Work out the finished part from the listing and answer in its coordinate system (mm). A direction names the side the tool comes from. Round coordinates to 2 decimals unless told otherwise and drop trailing zeros. Write each loop counter-clockwise with the first axis right and the second up, starting at its lowest first coordinate (ties: lowest second). Pieces come first, ordered by that corner, then holes. Notation, with made-up numbers: (70, 30) -> (85, 30) arc R21 ccw to (85, 51) -> close; hole circle Ø5 at (76.25, -16.5). An arc over 180 degrees is marked (long way). Answer as a JSON object with one key per item and string values. Group by question number.
from build123d import *

# Parameters (mm, degrees)
BOSS_EXTRUDE1_DEPTH = 5
SKETCH2_R           = 4
CUT_EXTRUDE1_DEPTH  = 5
CUT_EXTRUDE2_DEPTH  = 5
FILLET1_R           = 2


with BuildPart() as part:
    # Sketch1 → Boss-Extrude1 (new body)
    with BuildSketch(Plane.XY):
        with BuildLine():
            Line((-75, 0), (75, 0))
            ThreePointArc((75, 0), (0, 89.621051558), (-75, 0))
        make_face()
    extrude(amount=BOSS_EXTRUDE1_DEPTH)

    # Sketch2 → Cut-Extrude1 (cut)
    with BuildSketch(Plane.XY.offset(5)):
        with Locations((26.5, 8)):
            Circle(SKETCH2_R)
        with Locations((10, 80)):
            Circle(SKETCH2_R)
        with Locations((-10, 80)):
            Circle(SKETCH2_R)
        with Locations((-26.5, 8)):
            Circle(SKETCH2_R)
    extrude(amount=-CUT_EXTRUDE1_DEPTH, mode=Mode.SUBTRACT)

    # Sketch3 → Cut-Extrude2 (cut)
    with BuildSketch(Plane.XY.offset(5)):
        with BuildLine():
            Line((18.867867545, 5.996639034), (-18.867867545, 5.996639034))
            ThreePointArc((-18.867867545, 5.996639034), (-19.300154289, 6.245385832), (-19.302321259, 6.744126348))
            Line((-19.302321259, 6.744126348), (-10.267508213, 22.604365842))
            ThreePointArc((-10.267508213, 22.604365842), (-10.210571808, 22.944242288), (-10.387060948, 23.240231031))
            Line((-10.387060948, 23.240231031), (-43.118302779, 49.77907576))
            ThreePointArc((-43.118302779, 49.77907576), (-43.274670798, 50.334503122), (-42.8034018, 50.667453634))
            Line((-42.8034018, 50.667453634), (-18.945540234, 50.667453634))
            ThreePointArc((-18.945540234, 50.667453634), (-18.763089024, 50.70193075), (-18.605799379, 50.80060741))
            Line((-18.605799379, 50.80060741), (-1.358963418, 66.773116887))
            ThreePointArc((-1.358963418, 66.773116887), (0, 67.305731992), (1.358963418, 66.773116887))
            Line((1.358963418, 66.773116887), (18.605799379, 50.80060741))
            ThreePointArc((18.605799379, 50.80060741), (18.763089024, 50.70193075), (18.945540234, 50.667453634))
            Line((18.945540234, 50.667453634), (42.8034018, 50.667453634))
            ThreePointArc((42.8034018, 50.667453634), (43.274670798, 50.334503122), (43.118302779, 49.77907576))
            Line((43.118302779, 49.77907576), (10.387060948, 23.240231031))
            ThreePointArc((10.387060948, 23.240231031), (10.210571808, 22.944242288), (10.267508213, 22.604365842))
            Line((10.267508213, 22.604365842), (19.302321259, 6.744126348))
            ThreePointArc((19.302321259, 6.744126348), (19.300154289, 6.245385832), (18.867867545, 5.996639034))
        make_face()
    extrude(amount=-CUT_EXTRUDE2_DEPTH, mode=Mode.SUBTRACT)

    # Fillet1
    fillet1_edges = [part.edges().sort_by_distance(p)[0] for p in [
        (0, 89.621051558, 0),
        (0, 89.621051558, 5),
    ]]
    fillet(fillet1_edges, radius=FILLET1_R)


solid = part.part
1) Straight lines are drawn through the part: L1, parallel to Y at x = -13, z = 1.7; L2, parallel to X at y = 77.5, z = 1; L3, parallel to Y at x = -26.5, z = 2.1. For each, find the intervals that lie inside material, in ascending order.
2) A tool of negligible diameter and unlimited length cuts with its end or side. For faces 1 (the face through (31, 50.667, 3)), 2 (the face through (15, 25, 5)), from which of +Z, -Z, +X, -X, +Y, -Y can it reach the whole face along a straight path? Write none if from no direction.
3) A cutting plane is placed at A-A on z = 1.15. Determine the outline of the cut face in (x, y).
4) For a pull along Y with two mould halves and no side action, classify faces 3 (the face through (-14.85, 14.56, 2.54)), 4 (the face through (-1, 0, 2)), 5 (the face through (15, 25, 0)) as released by +Y, released by -Y, zero draft, split by the parting line, or undercut.
5) Each of these flat-tipped pins is pushed along its axis until it touches: P1, Ø1.5, axis at x = 6, z = 3, coming from the +Y side; P2, Ø1.5, axis at x = 7.5, z = 1, coming from the +Y side; P3, Ø2, axis at x = -19, z = 1.5, coming from the +Y side; P4, Ø1, axis at x = 21, y = 28, coming from the -Z side. Where does it stop, or does it pass through?
6) A cutting plane is placed at B-B on x = 26.5. State how many separate pieces and enclosed holes the cut face has, plus the area to 3 significant figures.
Established:
{
 "1": {"L1": "y = 0 to 6, 17.81 to 25.36, 55.99 to 77.35, 82.65 to 88.48", "L2": "x = -40.74 to -13.12, -6.88 to 6.88, 13.12 to 40.74", "L3": "y = 0 to 4, 12 to 36.3, 50.67 to 84.86"},
 "2": {"face 1": "+Z, -Z", "face 2": "+Z, +X, -X, +Y, -Y"},
 "3": {"outline": "(-74.81, 0) -> (74.81, 0) arc R76 ccw (long way) to start; hole (-43.12, 49.78) -> (-10.39, 23.24) arc R0.5 cw to (-10.27, 22.6) -> (-19.3, 6.74) arc R0.5 ccw to (-18.87, 6) -> (18.87, 6) arc R0.5 ccw to (19.3, 6.74) -> (10.27, 22.6) arc R0.5 cw to (10.39, 23.24) -> (43.12, 49.78) arc R0.5 ccw to (42.8, 50.67) -> (18.95, 50.67) arc R0.5 cw to (18.61, 50.8) -> (1.36, 66.77) arc R2 ccw to (-1.36, 66.77) -> (-18.61, 50.8) arc R0.5 cw to (-18.95, 50.67) -> (-42.8, 50.67) arc R0.5 ccw to start; hole circle Ø8 at (-26.5, 8); hole circle Ø8 at (-10, 80); hole circle Ø8 at (10, 80); hole circle Ø8 at (26.5, 8)"},
 "4": {"face 3": "undercut", "face 4": "released by -Y", "face 5": "zero draft"},
 "5": {"P1": "stops at y = 89.44", "P2": "stops at y = 89.26", "P3": "stops at y = 87.44", "P4": "stops at z = 0"},
 "6": {"separate pieces": "3", "enclosed holes": "0", "area": "311 mm²"}
}
